Here's the drawing with two shaded views (mm, measured from the low corner). I have some questions. A direction names the side the tool comes from. Coordinates: 2 decimals unless noted, no trailing zeros. Order: outer loops, then holes, each group sorted by start corner. A loop starts at its lowest first (then second) coordinate and runs counter-clockwise, first axis right, second up. Notation, with made-up numbers: (62.5, 26) - (112.5, 26) arc R19 ccw to (112.5, 48) - close; hole circle Ø2 at (31.25, 69). An arc over 180 degrees is marked (long way). Answer as a JSON object with one key per item and string values. Group by question number.
(1) Which directions (+Z, -Z, +X, -X, +Y, -Y) give clear straight access to the entire face, cutting with the end or side of a thin tool? Please do the marked faces 4, 5 and 6.
(2) Will these pins go through, and if not, where does the flat tip stop? P1, Ø2, axis at y = 4.5, z = 14, coming from the -X side; P2, Ø1, axis at x = 3.5, z = 12.5, coming from the +Y side; P3, Ø3, axis at x = 9, y = 9, coming from the -Z side; P4, Ø10.5, axis at x = 11, z = 11, coming from the +Y side.
(3) Please list where these lines run through material, in increasing order: probe 1 along X at (y, z) = (7.25, 11); probe 2 along Z at (x, y) = (5.25, 3.6); probe 3 along Z at (x, y) = (15.5, 2.25).
(4) Imagine slicing it at D-D, the plane z = 5.25. Write out the boundary of the cut face in (x, y), and give its area (3 significant figures).
(5) Imagine slicing it at A-A, the plane z = 11. Write out the boundary of the cut face in (x, y), and give its area (3 significant figures).
(6) We'd pull the mould along X, two halves only. Please class the marked faces 1, 2 and 3: pulls with the +X half, pulls with the -X half, needs draft (parallel to the pull), parting line crosses it, or undercut.
(7) Imagine slicing it at B-B, the plane x = 10. Write out the boundary of the cut face in (y, z).
(8) Imagine slicing it at C-C, the plane y = 9.5. Write out the boundary of the cut face in (x, z), and give its area (3 significant figures).
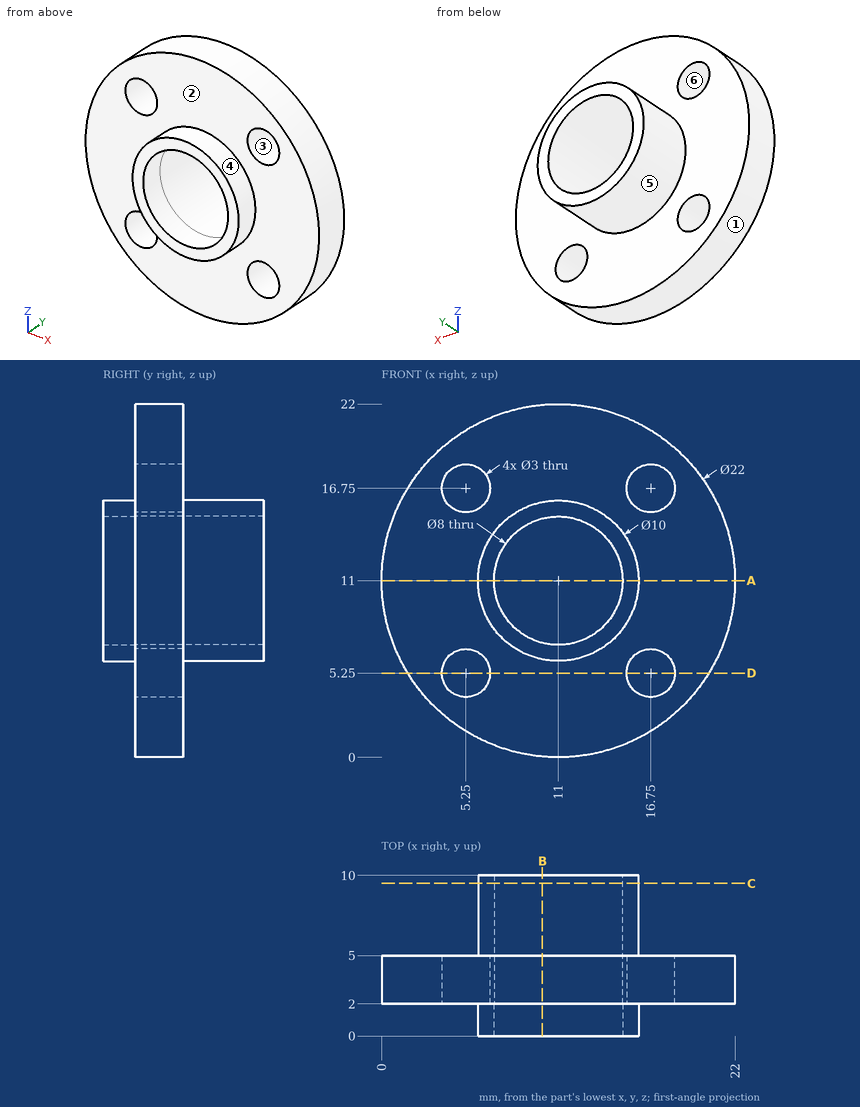
Result set:
{
 "1": {"face 4": "-Y", "face 5": "+Y", "face 6": "+Y, -Y"},
 "2": {"P1": "stops at x = 0.18", "P2": "stops at y = 5", "P3": "stops at z = 6.03", "P4": "stops at y = 10"},
 "3": {"probe 1": "x = 6 to 7, 15 to 16", "probe 2": "z = 1.62 to 3.75, 6.75 to 15.25, 18.25 to 20.38", "probe 3": "z = 0.96 to 4.42, 6.08 to 15.92, 17.58 to 21.04"},
 "4": {"outline": "(1.62, 2) - (3.75, 2) - (3.75, 5) - (1.62, 5) - close; (6.75, 2) - (15.25, 2) - (15.25, 5) - (6.75, 5) - close; (18.25, 2) - (20.38, 2) - (20.38, 5) - (18.25, 5) - close", "area": "38.3 mm^2"},
 "5": {"outline": "(0, 2) - (6, 2) - (6, 0) - (7, 0) - (7, 10) - (6, 10) - (6, 5) - (0, 5) - close; (15, 0) - (16, 0) - (16, 2) - (22, 2) - (22, 5) - (16, 5) - (16, 10) - (15, 10) - close", "area": "56.0 mm^2"},
 "6": {"face 1": "parting line crosses it", "face 2": "needs draft", "face 3": "undercut"},
 "7": {"outline": "(0, 6.1) - (2, 6.1) - (2, 0.05) - (5, 0.05) - (5, 6.1) - (10, 6.1) - (10, 7.13) - (0, 7.13) - close; (0, 14.87) - (10, 14.87) - (10, 15.9) - (5, 15.9) - (5, 21.95) - (2, 21.95) - (2, 15.9) - (0, 15.9) - close"},
 "8": {"outline": "circle Ø10 at (11, 11); hole circle Ø8 at (11, 11)", "area": "28.3 mm^2"}
}
